from build123d import *

# Parameters (mm, degrees)
CYLINDER003_R     = 3.7
CYLINDER003_DEPTH = 6
CYLINDER002_R     = 2.2
CYLINDER002_DEPTH = 70
CYLINDER_R        = 16
CYLINDER_DEPTH    = 100
BOX002_W          = 26
BOX002_H          = 6
BOX002_DEPTH      = 100
BOX001_W          = 38
BOX001_H          = 6
BOX001_DEPTH      = 112
CHAMFER_SIZE      = 3
CHAMFER001_SIZE   = 6
FILLET_R          = 1
FILLET001_R       = 1
FILLET002_R       = 1
BOX_W             = 22
BOX_H             = 52
BOX_DEPTH         = 30
CHAMFER002_SIZE   = 2
CHAMFER003_SIZE   = 4
CHAMFER004_SIZE   = 4
CHAMFER005_SIZE   = 4
CHAMFER006_SIZE   = 1


with BuildPart() as cylinder002:
    # Cylinder003 → Cylinder003 (new body)
    with BuildSketch(Plane(origin=(70, 0, 0), x_dir=(0, 0, -1), z_dir=(1, 0, 0))):
        Circle(CYLINDER003_R)
    extrude(amount=CYLINDER003_DEPTH)


with BuildPart() as obj1:
    # Cylinder002 → Cylinder002 (new body)
    with BuildSketch(Plane(origin=(0, 0, 0), x_dir=(0, 0, -1), z_dir=(1, 0, 0))):
        Circle(CYLINDER002_R)
    extrude(amount=CYLINDER002_DEPTH)

    # Fusion004: union Cylinder002
    add(cylinder002.part)


with BuildPart() as obj1_1:
    # Fusion004 placement: moved
    add(obj1.part.moved(Location((-53, -19, 15))))


with BuildPart() as tornillos:
    # Part__Mirroring: instance of obj1
    add(obj1_1.part.mirror(Plane(origin=(0, 0, 0), x_dir=(1, 0, 0), z_dir=(0, 1, 0))))

    # Fusion007: union obj1
    add(obj1_1.part)


with BuildPart() as obj2:
    # Cylinder → Cylinder (new body)
    with BuildSketch(Plane.XY):
        Circle(CYLINDER_R)
    extrude(amount=CYLINDER_DEPTH)


with BuildPart() as cube002:
    # Box002 → Box002 (new body)
    with BuildSketch(Plane(origin=(28, -3, -56), x_dir=(1, 0, 0), z_dir=(0, 0, 1))):
        with Locations((13, 3)):
            Rectangle(BOX002_W, BOX002_H)
    extrude(amount=BOX002_DEPTH)


with BuildPart() as fillet002:
    # Box001 → Box001 (new body)
    with BuildSketch(Plane(origin=(22, -3, -62), x_dir=(1, 0, 0), z_dir=(0, 0, 1))):
        with Locations((19, 3)):
            Rectangle(BOX001_W, BOX001_H)
    extrude(amount=BOX001_DEPTH)

    # Cut: cut Cube002
    add(cube002.part, mode=Mode.SUBTRACT)

    # Chamfer
    chamfer_edges = [fillet002.edges().sort_by_distance(p)[0] for p in [
        (22, 0, 50),
        (22, 0, -62),
        (60, 0, 50),
        (60, 0, -62),
    ]]
    chamfer(chamfer_edges, length=CHAMFER_SIZE)

    # Chamfer001
    chamfer001_edges = [fillet002.edges().sort_by_distance(p)[0] for p in [
        (54, 0, 44),
        (54, 0, -56),
        (28, 0, -56),
        (28, 0, 44),
    ]]
    chamfer(chamfer001_edges, length=CHAMFER001_SIZE)

    # Fillet
    fillet_edges = [fillet002.edges().sort_by_distance(p)[0] for p in [
        (54, -3, -6),
        (28, -3, -6),
        (54, 3, -6),
        (28, 3, -6),
    ]]
    fillet(fillet_edges, radius=FILLET_R)

    # Fillet001
    fillet001_edges = [fillet002.edges().sort_by_distance(p)[0] for p in [
        (41, -3, -56),
        (41, -3, 44),
        (41, 3, -56),
        (41, 3, 44),
    ]]
    fillet(fillet001_edges, radius=FILLET001_R)

    # Fillet002
    fillet002_edges = [fillet002.edges().sort_by_distance(p)[0] for p in [
        (31, -3, -53),
        (51, -3, -53),
        (31, -3, 41),
        (51, -3, 41),
        (31, 3, -53),
        (51, 3, -53),
        (31, 3, 41),
        (51, 3, 41),
    ]]
    fillet(fillet002_edges, radius=FILLET002_R)


with BuildPart() as obj3:
    # Box → Box (new body)
    with BuildSketch(Plane(origin=(0, -26, 0), x_dir=(1, 0, 0), z_dir=(0, 0, 1))):
        with Locations((11, 26)):
            Rectangle(BOX_W, BOX_H)
    extrude(amount=BOX_DEPTH)

    # Chamfer002
    chamfer002_edges = [obj3.edges().sort_by_distance(p)[0] for p in [
        (22, -26, 15),
        (22, 26, 15),
        (11, -26, 0),
        (11, -26, 30),
        (11, 26, 0),
        (11, 26, 30),
    ]]
    chamfer(chamfer002_edges, length=CHAMFER002_SIZE)

    # Fusion: union Fillet002
    add(fillet002.part)

    # Chamfer003
    chamfer003_edges = [obj3.edges().sort_by_distance(p)[0] for p in [
        (22, -3, 15),
        (22, 3, 15),
    ]]
    chamfer(chamfer003_edges, length=CHAMFER003_SIZE)

    # Chamfer004
    chamfer004_edges = [obj3.edges().sort_by_distance(p)[0] for p in [
        (22, 0, 0),
        (22, 0, 30),
    ]]
    chamfer(chamfer004_edges, length=CHAMFER004_SIZE)

    # Chamfer005
    chamfer005_edges = [obj3.edges().sort_by_distance(p)[0] for p in [
        (20, -3, 0),
        (24, -3, 0),
        (20, 3, 0),
        (24, 3, 0),
        (24, -3, 30),
        (20, -3, 30),
        (24, 3, 30),
        (20, 3, 30),
    ]]
    chamfer(chamfer005_edges, length=CHAMFER005_SIZE)

    # Cut001: cut obj2
    add(obj2.part, mode=Mode.SUBTRACT)

    # Cut002: cut tornillos
    add(tornillos.part, mode=Mode.SUBTRACT)

    # Chamfer006
    chamfer006_edges = [obj3.edges().sort_by_distance(p)[0] for p in [
        (22, -19, 18.7),
        (22, 19, 18.7),
    ]]
    chamfer(chamfer006_edges, length=CHAMFER006_SIZE)


solid = obj3.part
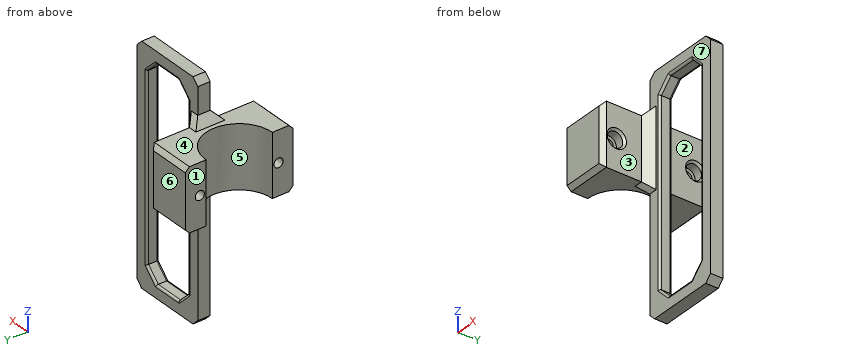
The listing builds one solid part. Answer for the finished solid, in the listing's coordinates (mm). Face numbers are marked on the shaded views. A direction names the side the tool comes from. Round coordinates to 2 decimals unless told otherwise and drop trailing zeros. Order: outer loops, then holes, each group sorted by start corner. A loop starts at its lowest first (then second) coordinate and runs counter-clockwise, first axis right, second up. Notation, with made-up numbers: (72.5, 81.5) - (117.5, 81.5) arc R7 ccw to (117.5, 89.5) - close; hole circle Ø4 at (74.5, 33.25). An arc over 180 degrees is marked (long way). Write item = value, one per line. Start each with the question number.
1) Section B-B, the plane y = 0 is taken. Write down the section's boundary in (x, z).
2) Section A-A, the plane z = 5 is taken. Write down the section's boundary in (x, y).
3) Straight lines are drawn through the part: L1, parallel to Y at x = 18.2, z = 15; L2, parallel to Z at x = 5, y = 19; L3, parallel to Z at x = 18.15, y = -19. For each, find the intervals that lie inside material, in ascending order.
4) For the marked faces 1, 2 and 3, determine the directions among +Z, -Z, +X, -X, +Y, -Y from which every point of the face is accessible in a straight line to the end or side of a thin tool.
5) For a pull along Y with two mould halves and no side action, classify the marked faces 4, 5, 6 and 7 as released by +Y, released by -Y, zero draft, split by the parting line, or undercut.
6) Section D-D, the plane y = 19 is taken. Write down the section's boundary in (x, z).
7) Section C-C, the plane x = 35.5 is taken. Write down the section's boundary in (y, z).
8) Given pin 1 (1.5 mm diameter, centred on x = 28.5, z = 9.5, fed in from +Y); pin 2 (1.5 mm diameter, centred on x = 22, y = 11.5, fed in from +Z); pin 3 (6 mm diameter, centred on y = 20.5, z = 16.5, fed in from +X), each flat-ended and moving along its own axis, determine where each tip first touches the part or whether it passes through.
Results list:
q1.outline = (16, 0) - (18, 0) - (22, -4) - (22, -59) - (25, -62) - (57, -62) - (60, -59) - (60, 47) - (57, 50) - (25, 50) - (22, 47) - (22, 34) - (18, 30) - (16, 30) - close; hole (28, -50) - (34, -56) - (48, -56) - (54, -50) - (54, 38) - (48, 44) - (34, 44) - (28, 38) - close
q2.outline = (0, -26) - (20, -26) - (22, -24) - (22, -7) - (26, -3) - (27, -3) arc R1 ccw to (28, -2) - (28, 2) arc R1 ccw to (27, 3) - (26, 3) - (22, 7) - (22, 24) - (20, 26) - (0, 26) - (0, 16) arc R16 cw to (0, -16) - close; (54, -2) arc R1 ccw to (55, -3) - (60, -3) - (60, 3) - (55, 3) arc R1 ccw to (54, 2) - close
q3.L1 = -26 to -22.7, -15.3 to 15.3, 22.7 to 26
q3.L2 = 0 to 12.8, 17.2 to 30
q3.L3 = 0 to 11.3, 18.7 to 30
q4.face_1 = +Z, -Z, -X, +Y, -Y
q4.face_2 = +Z, -Z, +X, +Y
q4.face_3 = +Z, -Z, +X, -Y
q5.face_4 = zero draft
q5.face_5 = undercut
q5.face_6 = released by +Y
q5.face_7 = released by -Y
q6.outline = (0, 0) - (22, 0) - (22, 10.3) - (21, 11.3) - (17, 11.3) - (17, 12.8) - (0, 12.8) - close; (0, 17.2) - (17, 17.2) - (17, 18.7) - (21, 18.7) - (22, 19.7) - (22, 30) - (0, 30) - close
q7.outline = (-3, -62) - (3, -62) - (3, -57) arc R1 ccw to (2, -56) - (-2, -56) arc R1 ccw to (-3, -57) - close; (-3, 45) arc R1 ccw to (-2, 44) - (2, 44) arc R1 ccw to (3, 45) - (3, 50) - (-3, 50) - close
q8.pin_1 = 2.66
q8.pin_2 = 30
q8.pin_3 = 22
